```python
from build123d import *

# Parameters (mm, degrees)
F0_W     = 38
F0_H     = 12
F1_DEPTH = 6
F2_R     = 4
F3_DEPTH = 5
F4_R     = 4
F5_DEPTH = 5
F6_R     = 3
F7_DEPTH = 5
F8_DEPTH = 5.5


with BuildPart() as f1:
    # F0 (on Top) → F1 (new body)
    with BuildSketch(Plane.XY):
        with Locations((19, 6)):
            Rectangle(F0_W, F0_H)
    extrude(amount=F1_DEPTH)

    # F2 (on face) → F3 (join)
    with BuildSketch(Plane.XY.offset(6)):
        with Locations((8, 6)):
            Circle(F2_R)
    extrude(amount=F3_DEPTH)

    # F4 (on face) → F5 (join)
    with BuildSketch(Plane.XY.offset(6)):
        with Locations((30, 6)):
            Circle(F4_R)
    extrude(amount=F5_DEPTH)

    # F6 (on face) → F7 (cut)
    with BuildSketch(Plane.XY):
        with Locations((28, 6)):
            Circle(F6_R)
    extrude(amount=F7_DEPTH, mode=Mode.SUBTRACT)

    # F6 (on face) → F8 (cut)
    with BuildSketch(Plane.XY):
        with Locations((28, 6)):
            Circle(F6_R)
        with Locations((11, 6)):
            Circle(F6_R)
    extrude(amount=F8_DEPTH, mode=Mode.SUBTRACT)


solid = f1.part
```
For this review, take the finished solid that the model builds, in its own axes (mm). A direction names the side the tool comes from. Round coordinates to 2 decimals unless told otherwise and drop trailing zeros. Write each loop counter-clockwise with the first axis right and the second up, starting at its lowest first coordinate (ties: lowest second). Pieces come first, ordered by that corner, then holes. Notation, with made-up numbers: (78.25, 17.25) -> (116.25, 17.25) arc R12 ccw to (116.25, 39.25) -> close; hole circle Ø1 at (82.5, -13.75). An arc over 180 degrees is marked (long way). One line per question, with ' | ' between items. Start each with the question number.
(1) Mouldability with a two-part tool opening along X and no side actions: class faces 4 (the face through (38, 6, 3)), 5 (the face through (0, 6, 3)), 6 (the face through (11, 6, 5.5)), 7 (the face through (8, 6, 11)) as released by +X, released by -X, zero draft, split by the parting line, or undercut.
(2) Tool access review of faces 1 (the face through (28, 6, 5.5)), 2 (the face through (26.8, 3.6, 8.5)), 3 (the face through (30, 6, 11)): name each direction out of +Z, -Z, +X, -X, +Y, -Y from which nothing blocks a thin tool from reaching the whole face with its end or side.
(3) Add section A-A, the plane y = 6. Write out the cut boundary in (x, z), plus the area to 3 significant figures.
(4) Add section B-B, the plane z = 5. Write out the cut boundary in (x, y), plus the area to 3 significant figures.
(5) Insertion check: P1, Ø1, axis at x = 26.5, z = 9.5, coming from the -Y side. The pin has a flat end and moves straight along its axis. Give the tip position at first contact, or say it passes through.
(6) Add section D-D, the plane z = 7. Write out the cut boundary in (x, y), plus the area to 3 significant figures.
(7) For line 1 along X through (y, z) = (4.75, 4); line 2 along Y through (x, z) = (28, 3.1); line 3 along X through (y, z) = (8.25, 2.75), list the stretches that pass through material, from the lowest coordinate up. Write a range as from..to.
(8) Add section C-C, the plane x = 8.5. Write out the cut boundary in (y, z), plus the area to 3 significant figures.
Answer list:
1) face 4: released by +X | face 5: released by -X | face 6: undercut | face 7: zero draft
2) face 1: -Z | face 2: +Z | face 3: +Z, +X, -X, +Y, -Y
3) outline: (0, 0) -> (8, 0) -> (8, 5.5) -> (14, 5.5) -> (14, 0) -> (25, 0) -> (25, 5.5) -> (31, 5.5) -> (31, 0) -> (38, 0) -> (38, 6) -> (34, 6) -> (34, 11) -> (26, 11) -> (26, 6) -> (12, 6) -> (12, 11) -> (4, 11) -> (4, 6) -> (0, 6) -> close | area: 242 mm²
4) outline: (0, 0) -> (38, 0) -> (38, 12) -> (0, 12) -> close; hole circle Ø6 at (11, 6); hole circle Ø6 at (28, 6) | area: 399 mm²
5) P1: y = 3.35
6) outline: circle Ø8 at (8, 6); circle Ø8 at (30, 6) | area: 101 mm²
7) line 1: 0..8.27, 13.73..25.27, 30.73..38 | line 2: 0..3, 9..12 | line 3: 0..9.02, 12.98..26.02, 29.98..38
8) outline: (0, 0) -> (4.34, 0) -> (4.34, 5.5) -> (7.66, 5.5) -> (7.66, 0) -> (12, 0) -> (12, 6) -> (9.97, 6) -> (9.97, 11) -> (2.03, 11) -> (2.03, 6) -> (0, 6) -> close | area: 93.4 mm²
